from build123d import *

# Parameters (mm, degrees)
BOSS_EXTRUDE1_DEPTH = 41.275
CUT_EXTRUDE1_REACH  = 330.685
SKETCH2_W           = 342.9
SKETCH2_H           = 28.575


with BuildPart() as part:
    # Sketch1 → Boss-Extrude1 (new body)
    with BuildSketch(Plane.XY):
        with BuildLine():
            Line((0, 19.05), (304.8, 19.05))
            ThreePointArc((304.8, 19.05), (323.85, 0), (304.8, -19.05))
            Line((304.8, -19.05), (0, -19.05))
            ThreePointArc((0, -19.05), (-19.05, 0), (0, 19.05))
        make_face()
        with BuildLine():
            Line((0, 6.43255), (304.8, 6.43255))
            ThreePointArc((304.8, 6.43255), (311.23255, 0), (304.8, -6.43255))
            Line((304.8, -6.43255), (0, -6.43255))
            ThreePointArc((0, -6.43255), (-6.43255, 0), (0, 6.43255))
        make_face(mode=Mode.SUBTRACT)
    extrude(amount=BOSS_EXTRUDE1_DEPTH)

    # Cut-Extrude1: up to this face of the body (flat: up to its plane)
    cut_extrude1_end = Plane(part.part.faces().sort_by_distance((152.4, 6.43255, 20.6375))[0])
    # Sketch2 → Cut-Extrude1 (cut, up to the picked face)
    with BuildSketch(Plane.XZ.offset(19.05), mode=Mode.PRIVATE) as cut_extrude1_sk1:
        with Locations((152.4, 20.6375)):
            Rectangle(SKETCH2_W, SKETCH2_H)
    cut_extrude1_tool1 = split(extrude(cut_extrude1_sk1.sketch, amount=-CUT_EXTRUDE1_REACH, mode=Mode.PRIVATE), bisect_by=cut_extrude1_end, keep=Keep.BOTH, mode=Mode.PRIVATE)
    add(cut_extrude1_tool1.solids().sort_by(Axis((152.4, -19.05, 20.6375), (0, 1, 0)))[0], mode=Mode.SUBTRACT)


solid = part.part
The listing builds one solid part. Answer for the finished solid, in the listing's coordinates (mm). A direction names the side the tool comes from. Give positions to 0.01 mm unless a question says otherwise; leave off trailing zeros. Order: outer loops, then holes, each group sorted by start corner. A loop starts at its lowest first (then second) coordinate and runs counter-clockwise, first axis right, second up. Notation, with made-up numbers: (70, 80) -> (85, 80) arc R20 ccw to (85, 96) -> close; hole circle Ø9 at (-34, 82.25). An arc over 180 degrees is marked (long way). Put each result on its own line as item: value.
Item 1: A cutting plane is placed at D-D on z = 12. Give the vertices of the cut face in (x, y).
Established:
outline: (-17.93, 6.43) -> (322.73, 6.43) arc R19.05 ccw to (304.8, 19.05) -> (0, 19.05) arc R19.05 ccw to start
Item 2: Given P1, Ø5, axis at x = 265, y = -2, coming from the -Z side; P2, Ø1, axis at x = 197.5, z = 32, coming from the -Y side, each flat-ended and moving along its own axis, determine where each tip first touches the part or whether it passes through.
Established:
P1: passes through
P2: stops at y = 6.43
Item 3: For faces 1 (the face through (319.12, 12.563, 20.349)), 2 (the face through (155, -6.433, 38)), 3 (the face through (150, -12, 34.925)), determine the directions among +Z, -Z, +X, -X, +Y, -Y from which every point of the face is accessible in a straight line to the end or side of a thin tool.
Established:
face 1: +Z, -Z, +X
face 2: +Z, -Z
face 3: +X, -X, -Y
Item 4: A cutting plane is placed at C-C on y = -16. Give the vertices of the cut face in (x, z) (3 decimals).
Established:
outline: (-10.339, 0) -> (315.139, 0) -> (315.139, 6.35) -> (-10.339, 6.35) -> close; (-10.339, 34.925) -> (315.139, 34.925) -> (315.139, 41.275) -> (-10.339, 41.275) -> close
Item 5: A cutting plane is placed at B-B on y = 0. Give the vertices of the cut face in (x, z) (3 decimals), plus the area to 3 significant figures.
Established:
outline: (-19.05, 0) -> (-6.433, 0) -> (-6.433, 6.35) -> (-19.05, 6.35) -> close; (-19.05, 34.925) -> (-6.433, 34.925) -> (-6.433, 41.275) -> (-19.05, 41.275) -> close; (311.233, 0) -> (323.85, 0) -> (323.85, 6.35) -> (311.233, 6.35) -> close; (311.233, 34.925) -> (323.85, 34.925) -> (323.85, 41.275) -> (311.233, 41.275) -> close
area: 320 mm^2
Item 6: A cutting plane is placed at A-A on x = 258. Give the vertices of the cut face in (y, z) (3 decimals), plus the area to 3 significant figures.
Established:
outline: (-19.05, 0) -> (-6.433, 0) -> (-6.433, 6.35) -> (-19.05, 6.35) -> close; (-19.05, 34.925) -> (-6.433, 34.925) -> (-6.433, 41.275) -> (-19.05, 41.275) -> close; (6.433, 0) -> (19.05, 0) -> (19.05, 41.275) -> (6.433, 41.275) -> close
area: 681 mm^2
Item 7: Straight lines are drawn through the part: line 1 (Z direction, x = 217, y = -16) (3 decimals); line 2 (Y direction, x = 171, z = 4); line 3 (Y direction, x = 171.5, z = 32.5). For each, find the intervals that lie inside material, in ascending order.
Established:
line 1: z = 0 to 6.35, 34.925 to 41.275
line 2: y = -19.05 to -6.43, 6.43 to 19.05
line 3: y = 6.43 to 19.05
Item 8: For a pull along Z with two mould halves and no side action, classify faces 4 (the face through (150, -12, 6.35)), 5 (the face through (155, 9, 41.275)), 6 (the face through (155, 9, 0)), 7 (the face through (-6.43, -0.14, 3.13)) as released by +Z, released by -Z, zero draft, split by the parting line, or undercut.
Established:
face 4: undercut
face 5: released by +Z
face 6: released by -Z
face 7: zero draft
